Autodesk Inventor part; units mm, degrees
ref_plane "Work Plane1" through (29, 0, 0) normal (0, -1, 0) x (1, 0, 0)
ref_plane "YZ Plane" through (0, 0, 0) normal (1, 0, 0) x (0, 1, 0)
ref_plane "XZ Plane" through (0, 0, 0) normal (0, 1, 0) x (-1, 0, 0)
sketch "Sketch1" plane through (0, 0, 0) normal (0, 0, 1) x (1, 0, 0)
  line L0 (-0.0931, 0) -> (7.9375, 0)
  line L1 (7.9375, 0) -> (7.9375, 2.0828)
  line L2 (7.9375, 2.0828) -> (1.5902, 2.0828)
  line L3 (1.5902, 2.0828) -> (0.0001, 2.0828)
  line L4 (0.0001, 2.0828) -> (0, 2.0828)
  line L5 (0, 2.0828) -> (0, 3.9624)
  line L6 (0, 3.9624) -> (-2.2098, 3.9624)
  line L7 (-2.2098, 3.9624) -> (-2.2098, 1.3785)
  line L8 (-2.2098, 1.3785) -> (-0.889, 1.3785)
  line L9 (-0.889, 1.3785) -> (-0.0931, 0)
  line L10 (-4.2393, 0) -> (9.967, 0)
  line L11 (0, -0.7925) -> (0, 4.7549)
  line L12 (1.5902, 2.0828) -> (0, 2.0828) construction
  dimension "d1" = 6.3473
  dimension "d2" = 1.5901
  dimension "d3" = 2.2098
  dimension "d4" = 1.3208
  dimension "d5" = 60
  dimension "d6" = 4.1656
  dimension "d7" = 4.1656
  dimension "d8" = 2.757
  dimension "d9" = 7.9248
  dimension "d26" = 7.9375
revolve "Body" add sketch "Sketch1" angle 360 about axis through (-0.0931, 0, 0) along (1, 0, 0)
sketch "Sketch2" plane through (-2.2098, 0, 0) normal (-1, 0, 0) x (0, 0, 1)
  circle A0 centre (0, 0) radius 1.3785
  line L0 (0, -5.5474) -> (0, 5.5474)
  line L1 (-5.5474, 0) -> (5.5474, 0)
  line L2 (1.3785, 0) -> (0.6892, -1.1938)
  line L3 (0.6892, -1.1938) -> (-0.6892, -1.1938)
  line L4 (-0.6892, -1.1938) -> (-1.3785, 0)
  line L5 (-1.3785, 0) -> (-0.6892, 1.1938)
  line L6 (-0.6892, 1.1938) -> (0.6892, 1.1938)
  line L7 (0.6892, 1.1938) -> (1.3785, 0)
extrude "Slot" add sketch "Sketch2" against normal up to next contours L7 A0 | A0 L2 | L6 L0 A0 | A0 L0 L3 | L0 L6 A0 | A0 L3 L0 | L4 A0 | A0 L5
fillet "Fillet1" radius 1.9558 1 edges at (-2.2098, -3.9624, 0)
thread "Thread"
chamfer "Chamfer1" distance 0.4869 distance2 0.4869 1 edges at (7.9375, -2.0828, 0) measured on face at (7.9375, -0.0837, 0.6892)
ref_plane "Work Plane1" through (29, 0, 0) normal (0, -1, 0) x (1, 0, 0)
fillet "Fillet2" radius 0.1 1 edges at (0.0001, -2.0828, 0)
equation "\"d30\" = R"
equation "\"d17\" = RR"
equation "\"d13\" = GEL"
equation "\"d15\" = -0.5 * SPD + 0.5 * GD"
equation "\"d16\" = GUL"
equation "\"d1\" = GEL"
equation "\"d3\" = KOH"
equation "\"d4\" = INTI"
equation "\"d6\" = GD"
equation "\"d7\" = BDM"
equation "\"d8\" = 1.1547 * SW"
equation "\"d9\" = KOD"
equation "\"d26\" = NLG"
equation "\"GD\" = NND"
equation "\"NLG\" = 7.9375"
equation "\"GEL\" = 6.34726"
equation "\"KOD\" = 7.9248"
equation "\"KOH\" = 2.2098"
equation "\"INTI\" = 1.3208"
equation "\"GAL\" = 1.59004"
equation "\"GUL\" = 0.48692"
equation "\"BDM\" = NND"
equation "\"SW\" = 2.3876"
equation "\"RR\" = 1.9558"
equation "\"SPD\" = 3.19176"
equation "\"R\" = 0.1"
equation "\"TOA\" = 30deg"
equation "\"GD1\" = SPD"
equation "\"THREADDIA\" = 4.1656"
equation "\"KOH1\" = 0.381"
equation "\"NND\" = 4.1656"
equation "\"E0\" = 2.75768"
properties part number "ANSI B18.3 - 8 - 32 x 5/16" material "Steel, Mild"
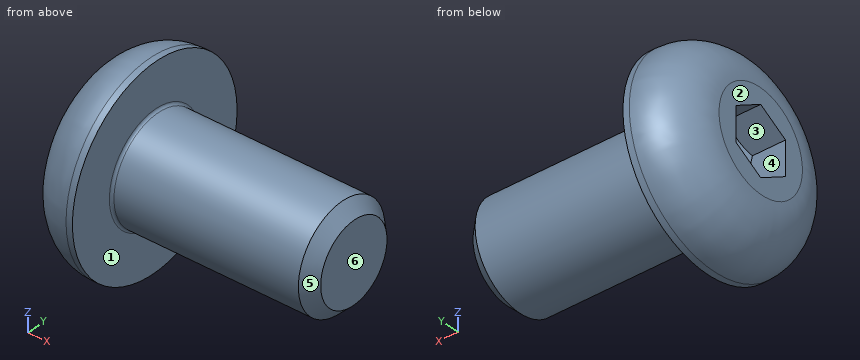
Part model, mm, in its own coordinate system. Face numbers are marked on the shaded views. A direction names the side the tool comes from. Give positions to 0.01 mm unless a question says otherwise; leave off trailing zeros. Write each loop counter-clockwise with the first axis right and the second up, starting at its lowest first coordinate (ties: lowest second). Pieces come first, ordered by that corner, then holes.
1) Which spindle directions (+Z, -Z, +X, -X, +Y, -Y) get a long thin tool onto all of the face, cutting with end or side? Do the marked faces 1, 2 and 3. Say none if no direction does.
Resolved:
face 1: +X
face 2: +Z, -Z, -X, +Y, -Y
face 3: -X
2) Probe L1, parallel to Z at x = -1.5, y = -0.75; L2, parallel to X at y = 2, z = -3; L3, parallel to Z at x = 3.5, y = -1. List the from-to ranges inside material, lowest first.
Resolved:
L1: z = -3.43 to -0.95, 0.95 to 3.43
L2: x = -1.38 to 0
L3: z = -1.83 to 1.83
3) Cut at A-A on x = 0.5. Write the cut outline in (y, z).
Resolved:
outline: circle Ø4.17 at (0, 0)
4) Pin check, flat tips, straight feed: pin 1 (4 mm diameter, centred on x = 5, z = -3, fed in from -Y); pin 2 (1.5 mm diameter, centred on x = -1.5, z = 0.5, fed in from -Y); pin 3 (3 mm diameter, centred on x = 4, y = 2.5, fed in from -Z). Stop position of each tip, or through.
Resolved:
pin 1: stops at y = -1.83
pin 2: stops at y = -3.88
pin 3: stops at z = -1.83
5) Two-plate mould, pull along Y, no slides. Class the marked faces 4, 5 and 6: released by +Y, released by -Y, zero draft, split by the parting line, or undercut.
Resolved:
face 4: undercut
face 5: split by the parting line
face 6: zero draft
